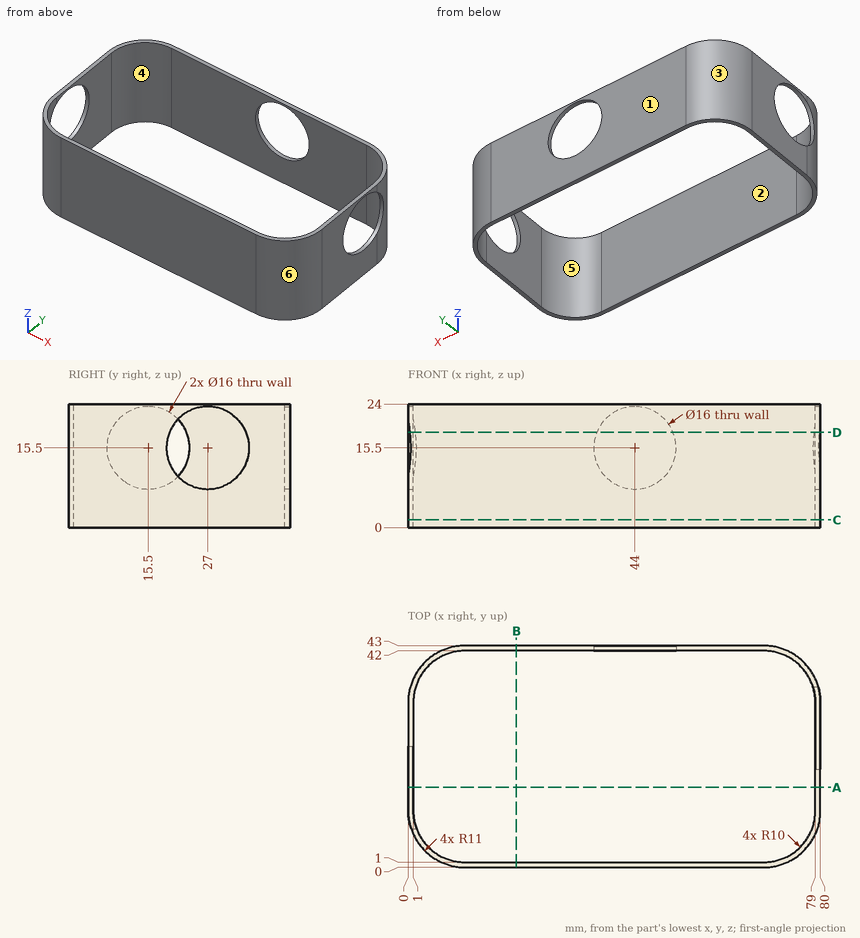
Print and shaded views of the part. All mm, measured from the part's lowest x, y and z. A direction names the side the tool comes from. Coordinates: 2 decimals unless noted, no trailing zeros. Write each loop counter-clockwise with the first axis right and the second up, starting at its lowest first coordinate (ties: lowest second). Pieces come first, ordered by that corner, then holes. Notation, with made-up numbers: (-2.5, 82.5) -> (3.5, 82.5) arc R6 cw to (3.5, 90.5) -> close; hole circle Ø6 at (-0.75, -11). An arc over 180 degrees is marked (long way). Use CSV: the item, a comma, the result in double quotes. Start each with the question number.
Q1. Cut at C-C, the plane z = 1.5. List the corners of the cut face in (x, y).
Q2. Pull direction X, two halves, no side cores. Call the marked faces 3, 4, 5 and 6: released by +X, released by -X, zero draft, split by the parting line, or undercut.
Q3. Cut at D-D, the plane z = 18.5. List the corners of the cut face in (x, y), then the cut area to 3 significant figures.
Q4. Drill centre lines: probe 1 along Y at (x, z) = (31, 14.75); probe 2 along X at (y, z) = (20, 2); probe 3 along X at (y, z) = (4, 5.25). Where is each one in solid material? Low to high.
Q5. 3-axis set-ups, long thin cutter, end or side, ignore diameter. For the marked faces 1 and 2: which of +Z, -Z, +X, -X, +Y, -Y reach the whole face in a straight line?
Q6. Cut at A-A, the plane y = 15.5. List the corners of the cut face in (x, z), then the cut area to 3 significant figures.
Q7. Cut at B-B, the plane x = 21. List the corners of the cut face in (y, z), then the cut area to 3 significant figures.
Checked values:
1,outline,"(0, 11) arc R11 ccw to (11, 0) -> (69, 0) arc R11 ccw to (80, 11) -> (80, 32) arc R11 ccw to (69, 43) -> (11, 43) arc R11 ccw to (0, 32) -> close; hole (1, 11) arc R10 ccw to (11, 1) -> (69, 1) arc R10 ccw to (79, 11) -> (79, 32) arc R10 ccw to (69, 42) -> (11, 42) arc R10 ccw to (1, 32) -> close"
2,face 3,"released by -X"
2,face 4,"undercut"
2,face 5,"undercut"
2,face 6,"released by +X"
3,outline,"(0, 22.92) -> (1, 22.92) -> (1, 32) arc R10 cw to (11, 42) -> (36.58, 42) -> (36.58, 43) -> (11, 43) arc R11 ccw to (0, 32) -> close; (0.39, 8.08) arc R11 ccw to (11, 0) -> (69, 0) arc R11 ccw to (80, 11) -> (80, 19.58) -> (79, 19.58) -> (79, 11) arc R10 cw to (69, 1) -> (11, 1) arc R10 cw to (1.43, 8.08) -> close; (51.42, 42) -> (69, 42) arc R10 cw to (78.7, 34.42) -> (79.73, 34.42) arc R11 ccw to (69, 43) -> (51.42, 43) -> close"
3,area,"179 mm²"
4,probe 1,"y = 0 to 1, 42 to 43"
4,probe 2,"x = 0 to 1, 79 to 80"
4,probe 3,"x = 2.51 to 3.86, 76.14 to 77.49"
5,face 1,"+Z, -Z, +X, -X, +Y"
5,face 2,"+Z, -Z"
6,outline,"(0, 0) -> (1, 0) -> (1, 7.5) -> (0, 7.5) -> close; (0, 23.5) -> (1, 23.5) -> (1, 24) -> (0, 24) -> close; (79, 0) -> (80, 0) -> (80, 24) -> (79, 24) -> close"
6,area,"32.0 mm²"
7,outline,"(0, 0) -> (1, 0) -> (1, 24) -> (0, 24) -> close; (42, 0) -> (43, 0) -> (43, 24) -> (42, 24) -> close"
7,area,"48.0 mm²"
